from build123d import *

# Parameters (mm, degrees)
SKETCH1_R               = 205
SKETCH1_R_2             = 8.425
SKETCH1_R_3             = 1.31
SKETCH1_R_4             = 3
BOSS_EXTRUDE1_DEPTH     = 2
SKETCH2_R               = 3
CUT_EXTRUDE1_DEPTH      = 1
CUT_EXTRUDE1_DEPTH_BACK = 3
SKETCH3_R               = 2.5
CUT_EXTRUDE2_DEPTH      = 10


with BuildPart() as part:
    # Sketch1 → Boss-Extrude1 (new body)
    with BuildSketch(Plane(origin=(0, 0, 0), x_dir=(1, 0, 0), z_dir=(0, 1, 0))):
        Circle(SKETCH1_R)
        with Locations((0, 140)):
            Circle(SKETCH1_R_2, mode=Mode.SUBTRACT)
        with Locations((0, -140)):
            Circle(SKETCH1_R_2, mode=Mode.SUBTRACT)
        with Locations((-13.2, 149.92)):
            Circle(SKETCH1_R_3, mode=Mode.SUBTRACT)
        with Locations((13.2, 149.92)):
            Circle(SKETCH1_R_3, mode=Mode.SUBTRACT)
        with Locations((13.2, 130.08)):
            Circle(SKETCH1_R_3, mode=Mode.SUBTRACT)
        with Locations((-13.2, 130.08)):
            Circle(SKETCH1_R_3, mode=Mode.SUBTRACT)
        with Locations((-13.2, -130.08)):
            Circle(SKETCH1_R_3, mode=Mode.SUBTRACT)
        with Locations((13.2, -130.08)):
            Circle(SKETCH1_R_3, mode=Mode.SUBTRACT)
        with Locations((13.2, -149.92)):
            Circle(SKETCH1_R_3, mode=Mode.SUBTRACT)
        with Locations((-13.2, -149.92)):
            Circle(SKETCH1_R_3, mode=Mode.SUBTRACT)
        with Locations((-82.5, 82.5)):
            Circle(SKETCH1_R_4, mode=Mode.SUBTRACT)
        with Locations((82.5, 82.5)):
            Circle(SKETCH1_R_4, mode=Mode.SUBTRACT)
        with Locations((82.5, -82.5)):
            Circle(SKETCH1_R_4, mode=Mode.SUBTRACT)
        with Locations((-82.5, -82.5)):
            Circle(SKETCH1_R_4, mode=Mode.SUBTRACT)
        with BuildLine():
            Line((-105, 45), (-105, -45))
            ThreePointArc((-105, -45), (-140, -80), (-175, -45))
            Line((-175, -45), (-175, 45))
            ThreePointArc((-175, 45), (-140, 80), (-105, 45))
        make_face(mode=Mode.SUBTRACT)
        with BuildLine():
            Line((175, 45), (175, -45))
            ThreePointArc((175, -45), (140, -80), (105, -45))
            Line((105, -45), (105, 45))
            ThreePointArc((105, 45), (140, 80), (175, 45))
        make_face(mode=Mode.SUBTRACT)
    extrude(amount=BOSS_EXTRUDE1_DEPTH)

    # Sketch2 → Cut-Extrude1 (cut, two sides)
    with BuildSketch(Plane(origin=(0, 2, 0), x_dir=(1, 0, 0), z_dir=(0, 1, 0))) as cut_extrude1_sk:
        with Locations((0, 192)):
            Circle(SKETCH2_R)
        with Locations((192, 0)):
            Circle(SKETCH2_R)
        with Locations((-192, 0)):
            Circle(SKETCH2_R)
    extrude(amount=CUT_EXTRUDE1_DEPTH, mode=Mode.SUBTRACT)
    extrude(cut_extrude1_sk.sketch, amount=-CUT_EXTRUDE1_DEPTH_BACK, mode=Mode.SUBTRACT)

    # Sketch3 → Cut-Extrude2 (cut)
    with BuildSketch(Plane(origin=(0, 2, 0), x_dir=(1, 0, 0), z_dir=(0, 1, 0))):
        with Locations((95, 15)):
            Circle(SKETCH3_R)
        with Locations((95, -15)):
            Circle(SKETCH3_R)
        with Locations((60, -15)):
            Circle(SKETCH3_R)
        with Locations((25, -15)):
            Circle(SKETCH3_R)
        with Locations((25, 15)):
            Circle(SKETCH3_R)
        with Locations((60, 15)):
            Circle(SKETCH3_R)
        with Locations((-60, 15)):
            Circle(SKETCH3_R)
        with Locations((-25, 15)):
            Circle(SKETCH3_R)
        with Locations((-25, -15)):
            Circle(SKETCH3_R)
        with Locations((-60, -15)):
            Circle(SKETCH3_R)
        with Locations((-95, -15)):
            Circle(SKETCH3_R)
        with Locations((-95, 15)):
            Circle(SKETCH3_R)
    extrude(amount=-CUT_EXTRUDE2_DEPTH, mode=Mode.SUBTRACT)


solid = part.part
Here's how the part is built. I have some questions about the finished solid (model axes, mm). A direction names the side the tool comes from. Coordinates: 2 decimals unless noted, no trailing zeros. Order: outer loops, then holes, each group sorted by start corner. A loop starts at its lowest first (then second) coordinate and runs counter-clockwise, first axis right, second up.
Item 1: For faces 5 (the face through (-3, 0, -3)), 6 (the face through (139.23, 0.99, -79.99)), which set-ups out of +Z, -Z, +X, -X, +Y, -Y let a thin tool reach every point of the face, with its end or its side?
Result sheet:
face 5: +Z, -Z, +X, -X, -Y
face 6: +Y, -Y
Item 2: If we section it at A-A on x = -144.5: List the corners of the cut face in (y, z) for me, plus the area to 3 significant figures.
Result sheet:
outline: (0, -145.41) - (2, -145.41) - (2, -79.71) - (0, -79.71) - close; (0, 79.71) - (2, 79.71) - (2, 145.41) - (0, 145.41) - close
area: 263 mm2
Item 3: If we section it at D-D on y = 0.9: State how many separate pieces and enclosed holes the cut face has, plus the area to 3 significant figures.
Result sheet:
separate pieces: 1
enclosed holes: 31
area: 111,000 mm2
Item 4: If we mould it in two halves opening along X, with no side actions, what happens to faces 1 (the face through (-3, 2, -3)), 2 (the face through (140.77, 0.99, 79.99)), 3 (the face through (-44.44, 0.986, 200.125)), 4 (the face through (-139.23, 0.99, 79.99))? For each: +X half, -X half, draft (parallel to the pull), parting line (faces both ways), or undercut.
Result sheet:
face 1: draft
face 2: undercut
face 3: parting line
face 4: undercut
Item 5: For P1, Ø3.5, axis at x = 13.2, z = 130.08, coming from the +Y side; P2, Ø2, axis at x = -13.2, z = 130.08, coming from the +Y side, each with a flat end and sliding along its axis, tell me the tip position at first contact or that it passes through.
Result sheet:
P1: stops at y = 2
P2: passes through
Item 6: If we section it at C-C on z = 123: List the corners of the cut face in (x, y) for me.
Result sheet:
outline: (-164, 0) - (164, 0) - (164, 2) - (-164, 2) - close
Item 7: I need wall thicknesses on line 1 (Z direction, x = 95, y = 1); line 2 (Z direction, x = 82.5, y = 1.5); line 3 (X direction, y = 1.3, z = 41). Which ranges of each line are inside material? Lowest first, please.
Result sheet:
line 1: z = -181.66 to -17.5, -12.5 to 12.5, 17.5 to 181.66
line 2: z = -187.67 to -85.5, -79.5 to 79.5, 85.5 to 187.67
line 3: x = -200.86 to -175, -105 to 105, 175 to 200.86
Item 8: If we section it at B-B on z = 38.5: List the corners of the cut face in (x, y) for me.
Result sheet:
outline: (-201.35, 0) - (-175, 0) - (-175, 2) - (-201.35, 2) - close; (-105, 0) - (105, 0) - (105, 2) - (-105, 2) - close; (175, 0) - (201.35, 0) - (201.35, 2) - (175, 2) - close
